```python
from build123d import *

# Parameters (mm, degrees)
SKETCH1_W                   = 101.6
SKETCH1_H                   = 50.8
BOSS_EXTRUDE1_DEPTH         = 5.08
H_0_266_DIAMETER_HOLE1_D    = 6.7564
SKETCH5_W                   = 8.255
SKETCH5_H                   = 12.7
BOSS_EXTRUDE2_DEPTH         = 12.7
SKETCH6_R                   = 1.5
CUT_EXTRUDE1_DEPTH          = 12.7
BOSS_EXTRUDE3_DEPTH         = 15.24
SKETCH9_W                   = 15.24
SKETCH9_H                   = 6.35
BOSS_EXTRUDE4_DEPTH         = 6.35
F_29_0_136_DIAMETER_HOLE1_D = 3.4544


with BuildPart() as part:
    # Sketch1 → Boss-Extrude1 (new body)
    with BuildSketch(Plane.XY):
        Rectangle(SKETCH1_W, SKETCH1_H)
    extrude(amount=BOSS_EXTRUDE1_DEPTH)

    # H _0.266_ Diameter Hole1 (through all)
    with Locations(Plane.XY.offset(5.08)):
        with Locations((38.1, 0), (-38.1, 0)):
            Hole(H_0_266_DIAMETER_HOLE1_D / 2)

    # Sketch5 → Boss-Extrude2 (add)
    with BuildSketch(Plane.XY.offset(5.08)):
        with Locations((-21.2725, 0)):
            Rectangle(SKETCH5_W, SKETCH5_H)
    boss_extrude2 = extrude(amount=BOSS_EXTRUDE2_DEPTH)

    # Sketch6 → Cut-Extrude1 (cut)
    with BuildSketch(Plane.ZY.offset(25.4)):
        with Locations((11.43, 0)):
            Circle(SKETCH6_R)
    cut_extrude1 = extrude(amount=-CUT_EXTRUDE1_DEPTH, mode=Mode.SUBTRACT)

    # Mirror1: Boss-Extrude2, Cut-Extrude1 across plane
    add(boss_extrude2.mirror(Plane(origin=(0, 0, 0), x_dir=(0, 0, 1), z_dir=(1, 0, 0))))
    add(cut_extrude1.mirror(Plane(origin=(0, 0, 0), x_dir=(0, 0, 1), z_dir=(1, 0, 0))), mode=Mode.SUBTRACT)

    # Sketch8 → Boss-Extrude3 (add)
    with BuildSketch(Plane.ZY.offset(-17.145)):
        with BuildLine():
            Line((11.43, 1.5), (11.43, 1.65))
            ThreePointArc((11.43, 1.65), (9.78, 0), (11.43, -1.65))
            Line((11.43, -1.65), (11.43, -1.5))
            ThreePointArc((11.43, -1.5), (9.93, 0), (11.43, 1.5))
        make_face()
        with BuildLine():
            Line((11.43, 1.65), (11.43, 6.35))
            Line((11.43, 6.35), (5.08, 6.35))
            Line((5.08, 6.35), (5.08, -6.35))
            Line((5.08, -6.35), (11.43, -6.35))
            Line((11.43, -6.35), (11.43, -1.65))
            ThreePointArc((11.43, -1.65), (9.78, 0), (11.43, 1.65))
        make_face()
    extrude(amount=BOSS_EXTRUDE3_DEPTH)

    # Sketch9 → Boss-Extrude4 (add)
    with BuildSketch(Plane(origin=(0, 6.35, 0), x_dir=(1, 0, 0), z_dir=(0, 1, 0))):
        with Locations((9.525, -8.255)):
            Rectangle(SKETCH9_W, SKETCH9_H)
    boss_extrude4 = extrude(amount=BOSS_EXTRUDE4_DEPTH)

    # Mirror2: Boss-Extrude4 across plane
    add(boss_extrude4.mirror(Plane.ZX))

    # 29 _0.136_ Diameter Hole1 (through all)
    with Locations(Plane.XY.offset(11.43)):
        with Locations((9.525, -7.62), (9.525, 7.62)):
            Hole(F_29_0_136_DIAMETER_HOLE1_D / 2)


solid = part.part
```
Read the model definition and answer for the solid it produces. Units are mm, in the model's axes. A direction names the side the tool comes from. Coordinates: 2 decimals unless noted, no trailing zeros. Write each loop counter-clockwise with the first axis right and the second up, starting at its lowest first coordinate (ties: lowest second). Pieces come first, ordered by that corner, then holes. Notation, with made-up numbers: (9.25, 77.5) -> (37.25, 77.5) arc R18 cw to (37.25, 82.5) -> close; hole circle Ø10 at (72, -9). An arc over 180 degrees is marked (long way). Write item = value, one per line.
(1) Section B-B on z = 6.75 is taken. Write down the section's boundary in (x, y) (3 decimals), plus the area to 3 significant figures.
From the geometry:
outline = (-25.4, -6.35) -> (-17.145, -6.35) -> (-17.145, 6.35) -> (-25.4, 6.35) -> close; (1.905, -12.7) -> (17.145, -12.7) -> (17.145, -6.35) -> (25.4, -6.35) -> (25.4, 6.35) -> (17.145, 6.35) -> (17.145, 12.7) -> (1.905, 12.7) -> close; hole circle Ø3.454 at (9.525, -7.62); hole circle Ø3.454 at (9.525, 7.62)
area = 578 mm2
(2) Which of the six approach directions +Z, -Z, +X, -X, +Y, -Y give full straight-line access (tool end or side, diameter ignored) to faces 4 (the face through (21, -6.35, 11)), 5 (the face through (17.145, 9, 8)), 6 (the face through (25.4, -2, 11)), 7 (the face through (17.145, 0, 15))?
From the geometry:
face_4 = +Z, +X, -Y
face_5 = +Z, +X, +Y
face_6 = +Z, +X, +Y, -Y
face_7 = +Z, +Y, -Y
(3) Given pin 1 Ø6 at (x, z) = (-21, 10.5) entering from -Y; pin 2 Ø4 at (y, z) = (-10.5, 11.5) entering from -X (3 decimals); pin 3 Ø12.5 at (x, y) = (6.5, -5) entering from +Z, each flat-ended and moving along its own axis, determine where each tip first touches the part or whether it passes through.
From the geometry:
pin_1 = -6.35
pin_2 = 1.905
pin_3 = 11.43
(4) Straight lines are drawn through the part: L1, parallel to Z at x = 23, y = 0; L2, parallel to Y at x = -21.75, z = 11.43; L3, parallel to Y at x = 38.1, z = 1.6. For each, find the intervals that lie inside material, in ascending order. Write a range as from..to.
From the geometry:
L1 = 0..9.93, 12.93..17.78
L2 = -6.35..-1.5, 1.5..6.35
L3 = -25.4..-3.38, 3.38..25.4
(5) For a pull along X with two mould halves and no side action, classify faces 1 (the face through (7.93, 6.96, 5.63)), 2 (the face through (9, -12.7, 8)), 3 (the face through (17.145, -9, 8)) as +X half, -X half, draft (parallel to the pull), parting line (faces both ways), or undercut.
From the geometry:
face_1 = undercut
face_2 = draft
face_3 = +X half
(6) Section C-C on y = 7.62 is taken. Write down the section's boundary in (x, z) (3 decimals).
From the geometry:
outline = (-50.8, 0) -> (7.798, 0) -> (7.798, 11.43) -> (1.905, 11.43) -> (1.905, 5.08) -> (-50.8, 5.08) -> close; (11.252, 0) -> (50.8, 0) -> (50.8, 5.08) -> (17.145, 5.08) -> (17.145, 11.43) -> (11.252, 11.43) -> close
(7) Section D-D on x = 38.1 is taken. Write down the section's boundary in (y, z), plus the area to 3 significant figures.
From the geometry:
outline = (-25.4, 0) -> (-3.38, 0) -> (-3.38, 5.08) -> (-25.4, 5.08) -> close; (3.38, 0) -> (25.4, 0) -> (25.4, 5.08) -> (3.38, 5.08) -> close
area = 224 mm2
(8) Section A-A on y = 0 is taken. Write down the section's boundary in (x, z) (3 decimals), plus the area to 3 significant figures.
From the geometry:
outline = (-50.8, 0) -> (-41.478, 0) -> (-41.478, 5.08) -> (-50.8, 5.08) -> close; (-34.722, 0) -> (34.722, 0) -> (34.722, 5.08) -> (25.4, 5.08) -> (25.4, 9.93) -> (1.905, 9.93) -> (1.905, 5.08) -> (-17.145, 5.08) -> (-17.145, 9.93) -> (-25.4, 9.93) -> (-25.4, 5.08) -> (-34.722, 5.08) -> close; (-25.4, 12.93) -> (-17.145, 12.93) -> (-17.145, 17.78) -> (-25.4, 17.78) -> close; (17.145, 12.93) -> (25.4, 12.93) -> (25.4, 17.78) -> (17.145, 17.78) -> close; (41.478, 0) -> (50.8, 0) -> (50.8, 5.08) -> (41.478, 5.08) -> close
area = 682 mm2
